from build123d import *

# Parameters (mm, degrees)
PAD_DEPTH       = 20
POCKET_DEPTH    = 33.001
SKETCH002_W     = 8.5
SKETCH002_H     = 8.5
POCKET001_DEPTH = 6
SKETCH003_R     = 3
POCKET002_DEPTH = 15.001
FILLET_R        = 10


with BuildPart() as part:
    # Sketch → Pad (new body)
    with BuildSketch(Plane.XY):
        with BuildLine():
            Line((-15, -14), (0, -14))
            Line((0, -14), (0, -8))
            ThreePointArc((0, -8), (8, 0), (0, 8))
            Line((0, 19), (0, 8))
            Line((-15, 19), (0, 19))
            Line((-15, 19), (-15, -14))
        make_face()
    extrude(amount=PAD_DEPTH)

    # Sketch001 → Pocket (cut, through all)
    with BuildSketch(Plane(origin=(0, 19, 0), x_dir=(-1, 0, 0), z_dir=(0, 1, 0))):
        with BuildLine():
            Line((19.016133, 20), (19.016133, 0))
            Line((19.016133, 0), (15.335206, 0))
            ThreePointArc((14.016133, 20), (13.069372, 9.894059), (15.335206, 0))
            Line((19.016133, 20), (14.016133, 20))
        make_face()
    extrude(amount=-POCKET_DEPTH, mode=Mode.SUBTRACT)

    # Sketch002 → Pocket001 (cut)
    with BuildSketch(Plane.YZ):
        with Locations((13, 10)):
            Rectangle(SKETCH002_W, SKETCH002_H)
    extrude(amount=-POCKET001_DEPTH, mode=Mode.SUBTRACT)

    # Sketch003 → Pocket002 (cut, through all)
    with BuildSketch(Plane.YZ):
        with Locations((13, 10)):
            Circle(SKETCH003_R)
    extrude(amount=-POCKET002_DEPTH, mode=Mode.SUBTRACT)

    # Fillet
    fillet_edges = [part.edges().sort_by_distance(p)[0] for p in [
        (-13.042214, -14, 10.356868),
    ]]
    fillet(fillet_edges, radius=FILLET_R)


solid = part.part
Geometry check sheet. Reference: the model listing, model coordinates, mm. A direction names the side the tool comes from. Round coordinates to 2 decimals unless told otherwise and drop trailing zeros. Loops run counter-clockwise (first coordinate to the right, second up) from the corner with the lowest first, then second, coordinate; pieces in that order, holes last. Notation, with made-up numbers: (1, -24) -> (58, -24) arc R24 cw to (58, 4) -> close; hole circle Ø8 at (32, 53). An arc over 180 degrees is marked (long way). Answer as a JSON object with one key per item and string values. Group by question number.
Item 1: Depth check by flat-ended pin: pin 1 Ø9.5 at (y, z) = (13, 10) entering from -X; pin 2 Ø1.8 at (y, z) = (-12, 12.5) entering from +X; pin 3 Ø12 at (y, z) = (12.5, 5.5) entering from +X. Enter the tip coordinate at first touch or a pass-through.
Item 2: Cross-section at D-D, the plane y = -8.5. Record the cut outline in (x, z).
Item 3: Set-up check for faces 1 (the face through (-3, 8.75, 10)), 2 (the face through (-6, 3, 0)), 3 (the face through (0, 14, 5)): record each of +Z, -Z, +X, -X, +Y, -Y from which the full face is reachable in a straight line by a thin tool's end or side.
Item 4: Release check for a two-part mould opening along Y. For faces 4 (the face through (-9.6, 10.6, 8.2)), 5 (the face through (0, -11, 10)), 6 (the face through (8, 0, 10)) record: pulls with the +Y half, pulls with the -Y half, needs draft (parallel to the pull), parting line crosses it, or undercut.
Item 5: Thickness scan on line 1 along Z through (x, y) = (-10.75, 13); line 2 along Z through (x, y) = (-1.75, 12); line 3 along Y through (x, z) = (-11, 10). Record the ranges inside material, lowest first.
Item 6: Cross-section at C-C, the plane y = 15. Record the cut outline in (x, z).
Item 7: Cross-section at B-B, the plane y = 0. Record the cut outline in (x, z), plus the area to 3 significant figures.
Item 8: Cross-section at A-A, the plane y = 10.5. Record the cut outline in (x, z).
Determined:
{
 "1": {"pin 1": "stops at x = -13.72", "pin 2": "stops at x = 0", "pin 3": "stops at x = 4.66"},
 "2": {"outline": "(-14.18, 0) -> (0, 0) -> (0, 20) -> (-12.91, 20) arc R33.07 cw to start"},
 "3": {"face 1": "+X", "face 2": "-Z, +X, -X, +Y, -Y", "face 3": "+Z, -Z, +X, +Y"},
 "4": {"face 4": "undercut", "face 5": "needs draft", "face 6": "parting line crosses it"},
 "5": {"line 1": "z = 0 to 7, 13 to 20", "line 2": "z = 0 to 5.75, 14.25 to 20", "line 3": "y = -10.08 to 10, 16 to 19"},
 "6": {"outline": "(-15, 0) -> (0, 0) -> (0, 5.75) -> (-6, 5.75) -> (-6, 7.76) -> (-13.28, 7.76) arc R32 cw to (-15, 0.86) -> close; (-14.02, 20) arc R32 cw to (-13, 12.24) -> (-6, 12.24) -> (-6, 14.25) -> (0, 14.25) -> (0, 20) -> close"},
 "7": {"outline": "(-15, 0) -> (8, 0) -> (8, 20) -> (-14.02, 20) arc R32 cw to (-15, 0.86) -> close", "area": "432 mm²"},
 "8": {"outline": "(-15, 0) -> (0, 0) -> (0, 5.75) -> (-6, 5.75) -> (-6, 8.34) -> (-13.21, 8.34) arc R32 cw to (-15, 0.86) -> close; (-14.02, 20) arc R32 cw to (-13, 11.66) -> (-6, 11.66) -> (-6, 14.25) -> (0, 14.25) -> (0, 20) -> close"}
}
